Check sheet for the modelled part. Datum: model origin and axes. Units: mm. Face numbers are marked on the shaded views. A direction names the side the tool comes from. Round coordinates to 2 decimals unless told otherwise and drop trailing zeros. Loops run counter-clockwise (first coordinate to the right, second up) from the corner with the lowest first, then second, coordinate; pieces in that order, holes last. Notation, with made-up numbers: (28.25, 43.25) -> (75.25, 43.25) arc R20 cw to (75.25, 82.25) -> close; hole circle Ø10 at (10.5, 23). An arc over 180 degrees is marked (long way). Return JSON: item names as keys, results as strings.
from build123d import *

# Parameters (mm, degrees)
CHANFREIN1_SIZE = 1


with BuildPart() as part:
    # Esquisse1 → Révolution1 (revolve)
    with BuildSketch(Plane.XY, mode=Mode.PRIVATE) as r_volution1_sk:
        Polygon((0, 13.75), (0, 22), (4.5, 22), (4.5, 17), (6, 17), (6, 18), (11.4, 18), (11.4, 13.75), align=None)
    revolve(r_volution1_sk.sketch.rotate(Axis((0, 0, 0), (1, 0, 0)), 90), axis=Axis((0, 0, 0), (1, 0, 0)))

    # Chanfrein1
    chanfrein1_edges = [part.edges().sort_by_distance(p)[0] for p in [
        (11.4, 0, -13.75),
        (11.4, 0, -18),
        (0, 0, -22),
        (0, 0, -13.75),
    ]]
    chamfer(chanfrein1_edges, length=CHANFREIN1_SIZE)

    # Esquisse3 → Diamètre du perçage Ø3.1 (3.1)1 (revolve, cut)
    with BuildSketch(Plane.ZX.offset(18.5)):
        Polygon((0, 0), (0, 4.431333959), (1.55, 3.5), (1.55, 0), align=None)
    diam_tre_du_per_age_3_1_3_1_1 = revolve(axis=Axis((-6.35, 18.5, 0), (1, 0, 0)), mode=Mode.SUBTRACT)

    # Symétrie1: Diamètre du perçage Ø3.1 (3.1)1 across plane
    add(diam_tre_du_per_age_3_1_3_1_1.mirror(Plane.ZX), mode=Mode.SUBTRACT)


solid = part.part
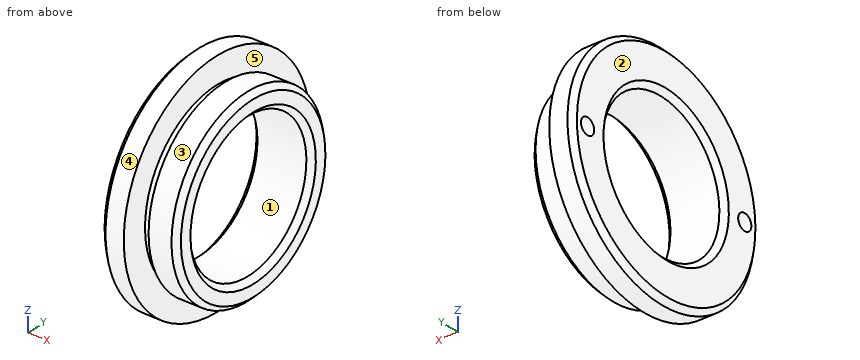
Q1. Section check A-A (y = 0). Record the boundary of the cut face in (x, z).
Results list:
{"outline": "(0, -21) -> (1, -22) -> (4.5, -22) -> (4.5, -17) -> (6, -17) -> (6, -18) -> (10.4, -18) -> (11.4, -17) -> (11.4, -14.75) -> (10.4, -13.75) -> (1, -13.75) -> (0, -14.75) -> close; (0, 14.75) -> (1, 13.75) -> (10.4, 13.75) -> (11.4, 14.75) -> (11.4, 17) -> (10.4, 18) -> (6, 18) -> (6, 17) -> (4.5, 17) -> (4.5, 22) -> (1, 22) -> (0, 21) -> close"}
Q2. Draft check along Z on the marked faces 1, 2 and 3. Enter one of: released by +Z, released by -Z, zero draft, split by the parting line, or undercut.
Results list:
{"face 1": "undercut", "face 2": "zero draft", "face 3": "split by the parting line"}
Q3. Go/stop test with flat-tipped pins: pin 1 (4 mm diameter, centred on x = 4, y = 5.5, fed in from +Z); pin 2 (8 mm diameter, centred on y = -13, z = -13, fed in from -X); pin 3 (3 mm diameter, centred on y = 18.5, z = 0, fed in from -X); pin 4 (2 mm diameter, centred on x = 3.5, z = 3, fed in from -Y). Record where each tip stops, or that it passes through.
Results list:
{"pin 1": "z = 21.72", "pin 2": "x = 0", "pin 3": "x = 3.53", "pin 4": "y = -21.91"}
Q4. Material ranges on line 1 (Y direction, x = 2.6, z = 0); line 2 (Y direction, x = 3.75, z = 0); line 3 (Y direction, x = 10.5, z = 11.5), recorded low to high.
Results list:
{"line 1": "-22 to -20.05, -16.95 to -13.75, 13.75 to 16.95, 20.05 to 22", "line 2": "-22 to -19.63, -17.37 to -13.75, 13.75 to 17.37, 19.63 to 22", "line 3": "-13.72 to -7.72, 7.72 to 13.72"}
Q5. Section check C-C (x = 8). Record the boundary of the cut face in (y, z).
Results list:
{"outline": "circle Ø36 at (0, 0); hole circle Ø27.5 at (0, 0)"}
Q6. Tool access check on the marked faces 4 and 5. Record the directions out of +Z, -Z, +X, -X, +Y, -Y that give a thin tool (end or side, any length) a straight path to the whole face; none if there is none.
Results list:
{"face 4": "+X, -X", "face 5": "none"}
Q7. Section check B-B (x = 2.5). Record the boundary of the cut face in (y, z).
Results list:
{"outline": "circle Ø44 at (0, 0); hole circle Ø3.1 at (-18.5, 0); hole circle Ø27.5 at (0, 0); hole circle Ø3.1 at (18.5, 0)"}
